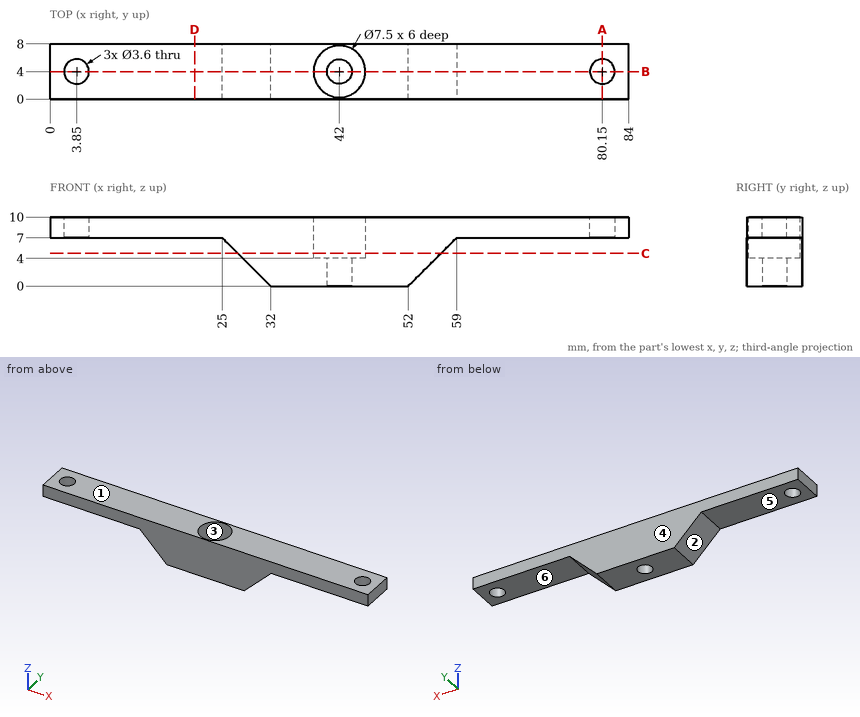
Study the drawing (mm; zero at the part's minimum x, y, z) and answer. A direction names the side the tool comes from. Round coordinates to 2 decimals unless told otherwise and drop trailing zeros. Order: outer loops, then holes, each group sorted by start corner. A loop starts at its lowest first (then second) coordinate and runs counter-clockwise, first axis right, second up. Notation, with made-up numbers: (88, 86) -> (140, 86) arc R30 ccw to (140, 117) -> close; hole circle Ø11 at (37.5, 75). An arc over 180 degrees is marked (long way). Answer as CSV lines item,"result". Start each with the question number.
(1) The part is cut by section C-C (z = 4.75). Determine the outline of the cut face in (x, y), then the cut area to 3 significant figures.
(2) Find the intervals of material crossed by probe 1 along X at (y, z) = (4.25, 9); probe 2 along Y at (x, z) = (3.85, 8.95); probe 3 along Z at (x, y) = (69, 5.25), in increasing order. Write a range as from..to.
(3) For a pull along X with two mould halves and no side action, classify the marked faces 1, 2 and 3 as +X half, -X half, draft (parallel to the pull), parting line (faces both ways), or undercut.
(4) Flat-ended cylindrical pins translate along their axes: pin 1 Ø6 at (x, z) = (13.5, 3) entering from -Y; pin 2 Ø2 at (y, z) = (7, 4) entering from +X; pin 3 Ø2 at (y, z) = (7, 5) entering from +X; pin 4 Ø4 at (x, y) = (73, 3.5) entering from -Z. Find the tip coordinate at first contact, or state that the pin passes through.
(5) The part is cut by section B-B (y = 4). Determine the outline of the cut face in (x, z).
(6) The part is cut by section D-D (x = 21). Determine the outline of the cut face in (y, z).
(7) A tool of negligible diameter and unlimited length cuts with its end or side. For the marked faces 4, 5 and 6, from which of +Z, -Z, +X, -X, +Y, -Y can it reach the whole face along a straight path? Write none if from no direction.
(8) The part is cut by section A-A (x = 80.15). Determine the outline of the cut face in (y, z).
Evaluation:
1,outline,"(27.25, 0) -> (56.75, 0) -> (56.75, 8) -> (27.25, 8) -> close; hole circle Ø7.5 at (42, 4)"
1,area,"192 mm²"
2,probe 1,"0..2.07, 5.63..38.26, 45.74..78.37, 81.93..84"
2,probe 2,"0..2.2, 5.8..8"
2,probe 3,"7..10"
3,face 1,"draft"
3,face 2,"-X half"
3,face 3,"undercut"
4,pin 1,"through"
4,pin 2,"x = 57"
4,pin 3,"x = 58"
4,pin 4,"z = 7"
5,outline,"(0, 7) -> (2.05, 7) -> (2.05, 10) -> (0, 10) -> close; (5.65, 7) -> (25, 7) -> (32, 0) -> (40.2, 0) -> (40.2, 4) -> (38.25, 4) -> (38.25, 10) -> (5.65, 10) -> close; (43.8, 0) -> (52, 0) -> (59, 7) -> (78.35, 7) -> (78.35, 10) -> (45.75, 10) -> (45.75, 4) -> (43.8, 4) -> close; (81.95, 7) -> (84, 7) -> (84, 10) -> (81.95, 10) -> close"
6,outline,"(0, 7) -> (8, 7) -> (8, 10) -> (0, 10) -> close"
7,face 4,"+Z, -Z, +X, -X, +Y"
7,face 5,"-Z, -X, +Y, -Y"
7,face 6,"-Z, +X, +Y, -Y"
8,outline,"(0, 7) -> (2.2, 7) -> (2.2, 10) -> (0, 10) -> close; (5.8, 7) -> (8, 7) -> (8, 10) -> (5.8, 10) -> close"
